Geometry: final body of the model. Coordinates: model frame, mm. A direction names the side the tool comes from. Coordinates: 2 decimals unless noted, no trailing zeros. Loops run counter-clockwise (first coordinate to the right, second up) from the corner with the lowest first, then second, coordinate; pieces in that order, holes last. Notation, with made-up numbers: M 73,34 L 114,34 A22 cw 114,63 Z; hole C -20.75,-5 d5. An arc over 180 degrees is marked long. Write item = value, one per line. Start each with the question number.
```python
from build123d import *

# Parameters (mm, degrees)
F0_R     = 27.78125
F0_R_2   = 3.96875
F0_R_3   = 2.15265
F0_R_4   = 11.1125
F1_DEPTH = 1.5875
F3_DEPTH = 1.5875
F4_COUNT = 6
F4_ANGLE = 300


with BuildPart() as f1:
    # F0 (on Top) → F1 (new body)
    with BuildSketch(Plane.XY):
        Circle(F0_R)
        with Locations((-12.3478521665, -12.3478521665)):
            Circle(F0_R_2, mode=Mode.SUBTRACT)
        with Locations((12.3478521665, -12.3478521665)):
            Circle(F0_R_3, mode=Mode.SUBTRACT)
        with Locations((-12.3478521665, 12.3478521665)):
            Circle(F0_R_3, mode=Mode.SUBTRACT)
        Circle(F0_R_4, mode=Mode.SUBTRACT)
        with Locations((12.3478521665, 12.3478521665)):
            Circle(F0_R_2, mode=Mode.SUBTRACT)
    extrude(amount=F1_DEPTH)

    # F2 (on face) → F3 (cut, through all)
    with BuildSketch(Plane.XY.offset(1.5875)):
        with BuildLine():
            Line((-3.0815642558, 11.5005543693), (-2.8761266387, 10.7338507446))
            ThreePointArc((-2.8761266387, 10.7338507446), (0, 11.1125), (2.8761266387, 10.7338507446))
            Line((2.8761266387, 10.7338507446), (3.0815642558, 11.5005543693))
            ThreePointArc((3.0815642558, 11.5005543693), (0, 11.90625), (-3.0815642558, 11.5005543693))
        make_face()
    f3 = extrude(amount=-F3_DEPTH, mode=Mode.SUBTRACT)

    # F4: F3 ×6 about axis
    f4_axis = Axis((0, 0, 0), (0, 0, -1))
    for i in range(1, F4_COUNT):
        add(f3.rotate(f4_axis, i * F4_ANGLE / (F4_COUNT - 1)), mode=Mode.SUBTRACT)


solid = f1.part
```
Item 1: Section query D-D (y = -19). Return the cut outline in (x, z).
Item 2: Line query: line 1 (Y direction, x = -9, z = 1.1); line 2 (Y direction, x = -12.5, z = 1.45); line 3 (X direction, y = -9.5, z = 1.1). Output: solid intervals per line, ascending. Write a range as from..to.
Item 3: Section query B-B (x = 0). Return the cut outline in (y, z).
Item 4: Pull-direction query (X, two-part tool) for faces 1 (the flat face through (12, 0, 1.588)), 2 (the cylindrical face through (-11.112, 0.041, 0.783)), 3 (the cylindrical face through (-5.521, 9.644, 0.783)); classes: released by +X, released by -X, zero draft, split by the parting line, or undercut.
Item 5: Reachability of faces 4 (the cylindrical face through (11.112, -0.041, 0.783)), 5 (the flat face through (12, 0, 0)) from +Z, -Z, +X, -X, +Y, -Y: full face, straight path, thin tool, end or side. Return the list, or none.
Item 6: Section query A-A (y = 0). Return the cut outline in (x, z), plus the area to 3 significant figures.
Item 7: Section query C-C (z = 0.45). Count the separate pieces of the cut face and the enclosed holes in it, plus the area to 3 significant figures.
Item 8: First-contact query: pin 1 (10 mm diameter, centred on x = -6, y = -11.5, fed in from -Z). Flat tip, straight axial feed; report the tip coordinate or a pass-through.
Verdict:
q1.outline = M -20.27,0 L 20.27,0 L 20.27,1.59 L -20.27,1.59 Z
q2.line_1 = -26.28..-14.48, -10.22..-7.79, 7.79..26.28
q2.line_2 = -24.81..-16.31, -8.38..10.2, 14.5..24.81
q2.line_3 = -26.11..-15.11, -9.58..-5.77, 5.77..26.11
q3.outline = M -27.78,0 L -11.91,0 L -11.91,1.59 L -27.78,1.59 Z; M 11.91,0 L 27.78,0 L 27.78,1.59 L 11.91,1.59 Z
q4.face_1 = zero draft
q4.face_2 = undercut
q4.face_3 = undercut
q5.face_4 = +Z, -Z
q5.face_5 = -Z, +X, -X, +Y, -Y
q6.outline = M -27.78,0 L -11.11,0 L -11.11,1.59 L -27.78,1.59 Z; M 11.11,0 L 27.78,0 L 27.78,1.59 L 11.11,1.59 Z
q6.area = 52.9 mm2
q7.separate_pieces = 1
q7.enclosed_holes = 5
q7.area = 1,880 mm2
q8.pin_1 = 0
